Read the model definition and answer for the solid it produces. Units are mm, in the model's axes. Face numbers are marked on the shaded views. A direction names the side the tool comes from. Give positions to 0.01 mm unless a question says otherwise; leave off trailing zeros. Order: outer loops, then holes, each group sorted by start corner. A loop starts at its lowest first (then second) coordinate and runs counter-clockwise, first axis right, second up. Notation, with made-up numbers: M -24.75,59 L 33.25,59 A22 ccw 33.25,92 Z; hole C 37,16 d6. An arc over 180 degrees is marked long. One line per item, written item: value.
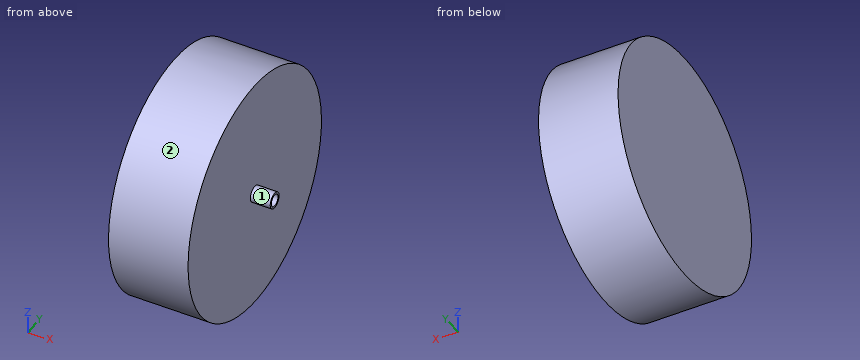
from build123d import *

# Parameters (mm, degrees)
SKETCH_1_R      = 4
SKETCH_1_R_2    = 3
EXTRUDE_1_DEPTH = 10
SKETCH_2_R      = 60
EXTRUDE_2_DEPTH = 40


with BuildPart() as part:
    # 草图1 → 凸台-拉伸1 (new body)
    with BuildSketch(Plane(origin=(0, 0, 0), x_dir=(0, 0, -1), z_dir=(1, 0, 0))):
        Circle(SKETCH_1_R)
        Circle(SKETCH_1_R_2, mode=Mode.SUBTRACT)
    extrude(amount=EXTRUDE_1_DEPTH)

    # 草图2 → 凸台-拉伸2 (add)
    with BuildSketch(Plane.ZY):
        Circle(SKETCH_2_R)
    extrude(amount=EXTRUDE_2_DEPTH)


solid = part.part
1) Find section C-C, the plane x = -10.5. Write down the section's boundary in (y, z).
Reported:
outline: C 0,0 d120
2) Consider probe 1 along X at (y, z) = (-36.5, 0.5); probe 2 along Y at (x, z) = (3.25, 0); probe 3 along Z at (x, y) = (-30, -4.5). Determine where each line is inside the solid, lowest interval first.
Reported:
probe 1: x = -40 to 0
probe 2: y = -4 to -3, 3 to 4
probe 3: z = -59.83 to 59.83
3) Each of these flat-tipped pins is pushed along its axis until it touches: pin 1 Ø6 at (x, z) = (0, -15.5) entering from -Y; pin 2 Ø6 at (x, y) = (-20, 12) entering from -Z; pin 3 Ø2 at (x, z) = (-27, 13.5) entering from +Y. Where does it stop, or does it pass through?
Reported:
pin 1: stops at y = -58.68
pin 2: stops at z = -59.32
pin 3: stops at y = 58.68
4) Which of the six approach directions +Z, -Z, +X, -X, +Y, -Y give full straight-line access (tool end or side, diameter ignored) to the marked faces 1 and 2?
Reported:
face 1: +X
face 2: +X, -X
5) Find section D-D, the plane z = -48. Write down the section's boundary in (x, y).
Reported:
outline: M -40,-36 L 0,-36 L 0,36 L -40,36 Z
6) Find section A-A, the plane y = 0. Write down the section's boundary in (x, z).
Reported:
outline: M -40,-60 L 0,-60 L 0,-4 L 10,-4 L 10,-3 L 0,-3 L 0,3 L 10,3 L 10,4 L 0,4 L 0,60 L -40,60 Z
